Geometry: final body of the model. Coordinates: model frame, mm. A direction names the side the tool comes from. Coordinates: 2 decimals unless noted, no trailing zeros. Answer in a Markdown table with one row per item.
from build123d import *

# Parameters (mm, degrees)
SKETCH_1_R               = 19
SKETCH_1_R_2             = 10
EXTRUDE_1_DEPTH          = 3
SKETCH_4_R               = 14
SKETCH_4_R_2             = 1.5000000000000007
SKETCH_4_R_3             = 1.4999999999999996
SKETCH_4_R_4             = 4.000000000000001
EXTRUDE_2_DEPTH          = 5
SKETCH_5_R               = 19
SKETCH_5_R_2             = 14
EXTRUDE_3_DEPTH          = 9
EXTRUDE_START            = -3
SKETCH_6_R               = 19
EXTRUDE_4_DEPTH          = 3
PATTERN_CIRCULAR_1_COUNT = 2
PATTERN_CIRCULAR_1_ANGLE = 90.0000000000002
PATTERN_CIRCULAR_2_COUNT = 2
PATTERN_CIRCULAR_2_ANGLE = 90.0000000000002
CHAMFER_1_SIZE           = 3
SKETCH_9_R               = 10.000000000000004
SKETCH_9_R_2             = 10.000000000000002
CUT_EXTRUDE_1_DEPTH      = 10
CUT_EXTRUDE_3_DEPTH      = 10
CUT_EXTRUDE_3_DEPTH_BACK = 10
SKETCH_13_W              = 150
SKETCH_13_H              = 9.999999999999996
CUT_EXTRUDE_5_DEPTH      = 37.000000000000014
FILLET_2_R               = 1
FILLET_3_R               = 3
CUT_EXTRUDE_6_DEPTH      = 3


with BuildPart() as part:
    # Sketch 1 → Extrude 1 (new body)
    with BuildSketch(Plane(origin=(0, 0, 0), x_dir=(1, 0, 0), z_dir=(0, 1, 0))):
        with Locations(Location((0, 0, 0), (0, 0, 270))):
            Circle(SKETCH_1_R)
        with Locations(Location((0, 0, 0), (0, 0, 270))):
            Circle(SKETCH_1_R_2, mode=Mode.SUBTRACT)
    extrude(amount=EXTRUDE_1_DEPTH)

    # Sketch 4 → Extrude 2 (add)
    with BuildSketch(Plane(origin=(0, 3, 0), x_dir=(1, 0, 0), z_dir=(0, 1, 0))):
        with Locations(Location((0, 0, 0), (0, 0, 270))):
            Circle(SKETCH_4_R)
        with Locations(Location((0, 7, 0), (0, 0, 270))):
            Circle(SKETCH_4_R_2, mode=Mode.SUBTRACT)
        with Locations(Location((7, 0, 0), (0, 0, 270))):
            Circle(SKETCH_4_R_3, mode=Mode.SUBTRACT)
        with Locations(Location((0, -7, 0), (0, 0, 90))):
            Circle(SKETCH_4_R_2, mode=Mode.SUBTRACT)
        with Locations(Location((-7, 0, 0), (0, 0, 90))):
            Circle(SKETCH_4_R_3, mode=Mode.SUBTRACT)
        with Locations(Location((0, 0, 0), (0, 0, 270))):
            Circle(SKETCH_4_R_4, mode=Mode.SUBTRACT)
    extrude(amount=EXTRUDE_2_DEPTH)

    # Sketch 5 → Extrude 3 (add)
    with BuildSketch(Plane(origin=(0, 3, 0), x_dir=(1, 0, 0), z_dir=(0, 1, 0))):
        with Locations(Location((0, 0, 0), (0, 0, 270))):
            Circle(SKETCH_5_R)
        with Locations(Location((0, 0, 0), (0, 0, 270))):
            Circle(SKETCH_5_R_2, mode=Mode.SUBTRACT)
    extrude(amount=EXTRUDE_3_DEPTH)

    # Sketch 6 → Extrude 4 (add)
    with BuildSketch(Plane(origin=(0, 12, 0), x_dir=(1, 0, 0), z_dir=(0, 1, 0)).offset(EXTRUDE_START)):
        with BuildLine():
            Line((-19.79898987322334, 73.85898987322332), (-73.85898987322334, 19.798989873223334))
            ThreePointArc((-73.85898987322332, 19.798989873223334), (-79.92862691031604, -10.715136106222507), (-54.06000000000001, -27.999999999999996))
            Line((-54.06, -28), (54.06, -28))
            ThreePointArc((54.06, -28.000000000000004), (79.92862691031604, -10.715136106222515), (73.85898987322334, 19.798989873223338))
            Line((73.85898987322334, 19.798989873223334), (19.79898987322334, 73.85898987322332))
            ThreePointArc((19.798989873223327, 73.85898987322332), (-1.19e-15, 82.05999999999999), (-19.798989873223327, 73.85898987322332))
        make_face()
        with Locations(Location((0, 0, 0), (0, 0, 270))):
            Circle(SKETCH_6_R, mode=Mode.SUBTRACT)
    extrude(amount=EXTRUDE_4_DEPTH)

    # Sketch 8 → Revolve 1 (revolve)
    with BuildSketch(Plane(origin=(0, 0, 0), x_dir=(0, 0, -1), z_dir=(1, 0, 0)), mode=Mode.PRIVATE) as revolve_1_sk:
        Polygon((82.06, 9), (80.06, 9.000000000000002), (85.09459778706366, 3.0000000000000018), (87.09459778706368, 3.0000000000000013), align=None)
    revolve_1 = revolve(revolve_1_sk.sketch.rotate(Axis((0, 9.000000000000002, -54.06), (0, -1, 0)), 45), axis=Axis((0, 9.000000000000002, -54.06), (0, -1, 0)))

    # Pattern Circular 1: Revolve 1 ×2 about axis
    pattern_circular_1_axis = Axis((0, -0.5999999999999999, 0), (0, 1, 0))
    for i in range(1, PATTERN_CIRCULAR_1_COUNT):
        add(revolve_1.rotate(pattern_circular_1_axis, i * PATTERN_CIRCULAR_1_ANGLE / (PATTERN_CIRCULAR_1_COUNT - 1)))

    # Pattern Circular 2: Revolve 1 ×2 about axis
    pattern_circular_2_axis = Axis((0, -0.5999999999999999, 0), (0, -1, 0))
    for i in range(1, PATTERN_CIRCULAR_2_COUNT):
        add(revolve_1.rotate(pattern_circular_2_axis, i * PATTERN_CIRCULAR_2_ANGLE / (PATTERN_CIRCULAR_2_COUNT - 1)))

    # Chamfer 1
    chamfer_1_edges = [part.edges().sort_by_distance(p)[0] for p in [
        (5.82e-15, 0, -19),
    ]]
    chamfer(chamfer_1_edges, length=CHAMFER_1_SIZE)

    # Sketch 9 → Cut-Extrude 1 (cut)
    with BuildSketch(Plane.XZ.offset(-9.000000000000002)):
        with Locations(Location((0, -54.06, 0), (0, 0, 270))):
            Circle(SKETCH_9_R)
        with Locations(Location((-54.06, 1.8875e-13, 0), (0, 0, 270))):
            Circle(SKETCH_9_R_2)
        with Locations(Location((54.06, 1.8875e-13, 0), (0, 0, 270))):
            Circle(SKETCH_9_R_2)
    extrude(amount=-CUT_EXTRUDE_1_DEPTH, mode=Mode.SUBTRACT)

    # Sketch 13 → Cut-Extrude 3 (cut, two sides: drawn at the far end of the back side and taken through both)
    with BuildSketch(Plane.XZ.offset(-9.000000000000002).offset(-CUT_EXTRUDE_3_DEPTH_BACK)):
        with Locations((0, 32)):
            Rectangle(SKETCH_13_W, SKETCH_13_H)
    extrude(amount=CUT_EXTRUDE_3_DEPTH + CUT_EXTRUDE_3_DEPTH_BACK, mode=Mode.SUBTRACT)

    # Sketch 14 → Cut-Extrude 5 (cut)
    with BuildSketch(Plane.XY):
        with BuildLine():
            Line((46.64380151290364, 9), (61.47619848709613, 9))
            add(Edge.make_bspline(
                [(80.11999999999978, 0), (73.17686755364808, 8.164120030068485), (61.47619848709613, 9)],
                knots=[0, 0, 0, 1, 1, 1], degree=2))
            Line((80.11999999999978, 0), (28, 0))
            add(Edge.make_bspline(
                [(28, 0), (34.94313244635168, 8.164120030068489), (46.64380151290364, 9)],
                knots=[0, 0, 0, 1, 1, 1], degree=2))
        make_face()
        with BuildLine():
            Line((-46.64380151290364, 9), (-61.47619848709613, 9))
            add(Edge.make_bspline(
                [(-80.11999999999978, 0), (-73.1768675536481, 8.164120030068485), (-61.47619848709613, 9)],
                knots=[0, 0, 0, 1, 1, 1], degree=2))
            Line((-80.11999999999978, 0), (-28, 0))
            add(Edge.make_bspline(
                [(-28, 0), (-34.94313244635168, 8.164120030068489), (-46.64380151290364, 9)],
                knots=[0, 0, 0, 1, 1, 1], degree=2))
        make_face()
    extrude(amount=CUT_EXTRUDE_5_DEPTH, mode=Mode.SUBTRACT)

    # Fillet 2
    # the kernel refuses this fillet: 1 mm, written as the material it takes off along each edge
    with BuildSketch(Plane(origin=(54.06, 3.0000000000000018, 1.9206e-13), x_dir=(-0.7172935619885054, 0, 0.6967710857446958), z_dir=(0.6967710857446958, 0, 0.7172935619885054))) as fillet_2_piece_1:
        with BuildLine():
            CenterArc((31.034597787063664 + FILLET_2_R * 0.466307658155, -FILLET_2_R), FILLET_2_R, 90, 49.99999999999997)
            Line((31.034597787063664 - FILLET_2_R * 0.299736784964, -FILLET_2_R * 0.357212390313), (31.034597787063664, 0))
            Line((31.034597787063664, 0), (31.034597787063664 + FILLET_2_R * 0.466307658155, 0))
        make_face()
    revolve(axis=Axis((54.06, 3.0000000000000018, 1.9206e-13), (0, -1, 0)), revolution_arc=268.3370368114634, mode=Mode.SUBTRACT)
    with BuildSketch(Plane(origin=(0, 3.0000000000000018, -54.06), x_dir=(0.7071067811865477, 0, -0.7071067811865475), z_dir=(-0.7071067811865475, 0, -0.7071067811865477))) as fillet_2_piece_2:
        with BuildLine():
            CenterArc((31.03459778706366 + FILLET_2_R * 0.466307658155, -FILLET_2_R), FILLET_2_R, 89.99999999999939, 50.00000000000074)
            Line((31.03459778706366 + FILLET_2_R * 0.466307658155, 0), (31.03459778706366, 0))
            Line((31.03459778706366, 0), (31.03459778706366 - FILLET_2_R * 0.299736784964, -FILLET_2_R * 0.357212390313))
        make_face()
    revolve(axis=Axis((0, 3.0000000000000018, -54.06), (0, -1, 0)), mode=Mode.SUBTRACT)
    with BuildSketch(Plane(origin=(-54.06, 3.0000000000000018, 1.9206e-13), x_dir=(0.7172935619885052, 0, 0.6967710857446959), z_dir=(-0.6967710857446959, 0, 0.7172935619885052))) as fillet_2_piece_3:
        with BuildLine():
            CenterArc((31.034597787063667 + FILLET_2_R * 0.466307658155, FILLET_2_R), FILLET_2_R, 219.99999999999983, 50.00000000000017)
            Line((31.034597787063667 - FILLET_2_R * 0.299736784964, FILLET_2_R * 0.357212390313), (31.034597787063667, 0))
            Line((31.034597787063667, 0), (31.034597787063667 + FILLET_2_R * 0.466307658155, 0))
        make_face()
    revolve(axis=Axis((-54.06, 3.0000000000000018, 1.9206e-13), (0, 1, 0)), revolution_arc=268.3370368114635, mode=Mode.SUBTRACT)

    # Fillet 3
    fillet_3_edges = [part.edges().sort_by_distance(p)[0] for p in [
        (4.29e-15, 12, -14),
        (5.82e-15, 9, -19),
    ]]
    fillet(fillet_3_edges, radius=FILLET_3_R)

    # Sketch 15 → Cut-Extrude 6 (cut)
    with BuildSketch(Plane(origin=(0, 12, 0), x_dir=(1, 0, 0), z_dir=(0, 1, 0))):
        with BuildLine():
            Line((-69.81557659130944, 23.146529032997286), (-70.76615831998882, 22.89182142645786))
            Line((-70.76615831998882, 22.89182142645786), (-22.89182142645785, 70.7661583199888))
            Line((-22.89182142645785, 70.7661583199888), (-23.14652903299728, 69.81557659130941))
            add(Edge.make_bspline(
                [(-23.14652903299728, 69.81557659130941), (-27.520231774406998, 52.52739820941615), (-39.75792206135788, 39.75792206135787)],
                knots=[0, 0, 0, 1, 1, 1], degree=2))
            add(Edge.make_bspline(
                [(-69.81557659130944, 23.146529032997286), (-52.52739820941618, 27.52023177440699), (-39.75792206135788, 39.75792206135787)],
                knots=[0, 0, 0, 1, 1, 1], degree=2))
        make_face()
        with BuildLine():
            Line((70.76615831998882, 22.89182142645786), (22.89182142645785, 70.7661583199888))
            Line((22.89182142645785, 70.7661583199888), (23.14652903299728, 69.81557659130941))
            add(Edge.make_bspline(
                [(23.14652903299728, 69.81557659130941), (27.520231774406998, 52.52739820941615), (39.75792206135788, 39.75792206135787)],
                knots=[0, 0, 0, 1, 1, 1], degree=2))
            add(Edge.make_bspline(
                [(69.81557659130944, 23.146529032997286), (52.52739820941618, 27.52023177440699), (39.75792206135788, 39.75792206135787)],
                knots=[0, 0, 0, 1, 1, 1], degree=2))
            Line((69.81557659130944, 23.146529032997286), (70.76615831998882, 22.89182142645786))
        make_face()
    extrude(amount=-CUT_EXTRUDE_6_DEPTH, mode=Mode.SUBTRACT)


solid = part.part
(1) First-contact query: pin 1 Ø2 at (x, y) = (4, 6.5) entering from +Z; pin 2 Ø4 at (x, z) = (-7, 0) entering from +Y; pin 3 Ø16 at (x, z) = (-54.06, 0) entering from +Y; pin 4 Ø1 at (x, z) = (-37, 4) entering from -Y. Flat tips, straight axial feed; report the tip coordinate or a pass-through.
Verdict:
| item | result |
|---|---|
| pin 1 | stops at z = 19.02 |
| pin 2 | stops at y = 8 |
| pin 3 | passes through |
| pin 4 | stops at y = 9 |
(2) Access query for faces 4 (the face through (-9.76, 1.48, -2.17)), 5 (the face through (63, 9, -26)), 6 (the face through (-31, 3, -61)), 7 (the face through (-81.23, 10.48, 6.77)). Directions: +Z, -Z, +X, -X, +Y, -Y. A direction counts if a zero-diameter tool reaches every point of the face in a straight line with its end or side. Return the directions, or none.
Verdict:
| item | result |
|---|---|
| face 4 | -Y |
| face 5 | -Z, +X, +Y |
| face 6 | -Z, +X, -X, -Y |
| face 7 | -X, +Y |
(3) Pull-direction query (Z, two-part tool) for faces 1 (the face through (-10.4, 0, -0.2)), 2 (the face through (25.05, 8.71, -67.11)), 3 (the face through (81.02, 10.48, 7.56)); classes: pulls with the +Z half, pulls with the -Z half, needs draft (parallel to the pull), parting line crosses it, or undercut.
Verdict:
| item | result |
|---|---|
| face 1 | needs draft |
| face 2 | undercut |
| face 3 | parting line crosses it |
(4) Ray query, probe 1 along X at (y, z) = (6.5, -7.5); probe 2 along Z at (x, y) = (-17.5, 6.5); probe 3 along Z at (x, y) = (-2, 7). Return the intervals inside material, ascending.
Verdict:
| item | result |
|---|---|
| probe 1 | x = -83.21 to -81.14, -26.98 to -24.91, -17.5 to -1.41, 1.41 to 17.5, 24.91 to 26.98, 81.14 to 83.21 |
| probe 2 | z = -78.55 to -76.04, -32.08 to -29.57, -7.51 to 7.51 |
| probe 3 | z = -83.67 to -81.67, -26.45 to -24.45, -19.07 to -3.46, 3.46 to 19.07 |
